Read the model definition and answer for the solid it produces. Units are mm, in the model's axes. Face numbers are marked on the shaded views. Coordinates: 2 decimals unless noted, no trailing zeros. Loops run counter-clockwise (first coordinate to the right, second up) from the corner with the lowest first, then second, coordinate; pieces in that order, holes last.
Q1. Straight lines are drawn through the part: line 1 (Y direction, x = -46.5, z = 291.5); line 2 (X direction, y = -29, z = 473); line 3 (Y direction, x = -1.1, z = 250). For each, find the intervals that lie inside material, in ascending order.
Q2. Section C-C (z = 407) is taken. Give the vertices of the cut face in (x, y), then the cut area to 3 significant figures.
Q3. Section B-B (x = -26) is taken. Give the vertices of the cut face in (y, z), then the cut area to 3 significant figures.
Q4. The mould has two halves that part along Y. Classify the marked faces 1, 2 and 3: pulls with the +Y half, pulls with the -Y half, needs draft (parallel to the pull), parting line crosses it, or undercut.
Q5. Flat-ended cylindrical pins translate along their axes: P1, Ø2, axis at x = -1, z = 361.5, coming from the +Y side; P2, Ø1.6, axis at x = -1, y = -22, coming from the -Z side; P3, Ø5.5, axis at y = 15, z = 191.5, coming from the +X side; P4, Ø1.5, axis at x = -40, z = 116.5, coming from the +Y side. Find the tip coordinate at first contact, or state that the pin passes through.
Q6. Section A-A (z = 250) is taken. Give the vertices of the cut face in (x, y), then the cut area to 3 significant figures.
from build123d import *

# Parameters (mm, degrees)
BOSS_EXTRUDE1_DEPTH = 500
SKETCH2_R           = 12.5
CUT_EXTRUDE1_DEPTH  = 54.301270189
SKETCH3_W           = 60
SKETCH3_H           = 10
CUT_EXTRUDE2_DEPTH  = 2
SKETCH4_W           = 500
SKETCH4_H           = 20
BOSS_EXTRUDE2_DEPTH = 2


with BuildPart() as part:
    # Sketch1 → Boss-Extrude1 (new body)
    with BuildSketch(Plane.XY):
        Polygon((0, 0), (-43.301270189, 25), (-53.301270189, 25), (-53.301270189, 23), (-43.837168574, 23), (-2, -1.154700538), (-2, -48), (-50, -48), (-50, -50), (0, -50), align=None)
    extrude(amount=BOSS_EXTRUDE1_DEPTH)

    # Sketch2 → Cut-Extrude1 (cut, through all)
    with BuildSketch(Plane(origin=(0, 0, 0), x_dir=(0, 0, -1), z_dir=(1, 0, 0))):
        with Locations((-250, -27)):
            Circle(SKETCH2_R)
    extrude(amount=-CUT_EXTRUDE1_DEPTH, mode=Mode.SUBTRACT)

    # Sketch3 → Cut-Extrude2 (cut)
    with BuildSketch(Plane(origin=(0, 0, 0), x_dir=(0, 0, -1), z_dir=(1, 0, 0))):
        with Locations((-140, -22.5)):
            Rectangle(SKETCH3_W, SKETCH3_H)
        with Locations((-360, -22.5)):
            Rectangle(SKETCH3_W, SKETCH3_H)
    extrude(amount=-CUT_EXTRUDE2_DEPTH, mode=Mode.SUBTRACT)

    # Sketch4 → Boss-Extrude2 (add)
    with BuildSketch(Plane.ZY.offset(53.301270189)):
        with Locations((250, 15)):
            Rectangle(SKETCH4_W, SKETCH4_H)
    extrude(amount=-BOSS_EXTRUDE2_DEPTH)


solid = part.part
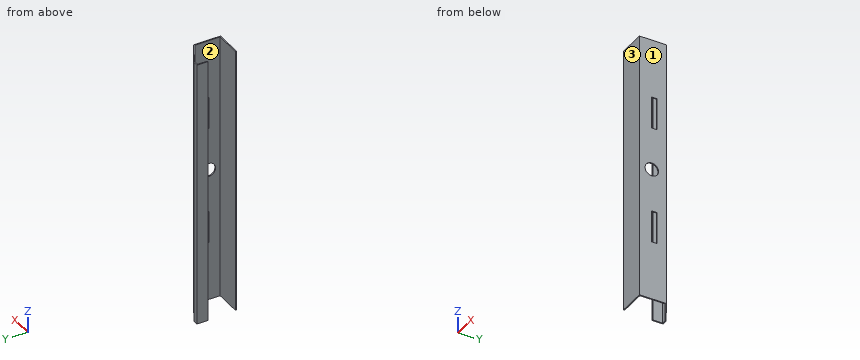
Numbers:
1. line 1: y = -50 to -48, 23 to 25
1. line 2: x = -2 to 0
1. line 3: y = -50 to -39.5, -14.5 to 0.64
2. outline: (-53.3, 5) - (-51.3, 5) - (-51.3, 23) - (-43.84, 23) - (-2, -1.15) - (-2, -48) - (-50, -48) - (-50, -50) - (0, -50) - (0, 0) - (-43.3, 25) - (-53.3, 25) - close
2. area: 349 mm2
3. outline: (-50, 0) - (-48, 0) - (-48, 500) - (-50, 500) - close; (12.7, 0) - (15.01, 0) - (15.01, 500) - (12.7, 500) - close
3. area: 2,150 mm2
4. face 1: needs draft
4. face 2: undercut
4. face 3: pulls with the -Y half
5. P1: stops at y = 1.15
5. P2: stops at z = 0
5. P3: stops at x = -21.22
5. P4: stops at y = 23.53
6. outline: (-53.3, 5) - (-51.3, 5) - (-51.3, 23) - (-43.84, 23) - (-2, -1.15) - (-2, -14.5) - (0, -14.5) - (0, 0) - (-43.3, 25) - (-53.3, 25) - close; (-50, -50) - (0, -50) - (0, -39.5) - (-2, -39.5) - (-2, -48) - (-50, -48) - close
6. area: 299 mm2
